Geometry: final body of the model. Coordinates: model frame, mm. Coordinates: 2 decimals unless noted, no trailing zeros. Write each loop counter-clockwise with the first axis right and the second up, starting at its lowest first coordinate (ties: lowest second). Pieces come first, ordered by that corner, then holes. Notation, with made-up numbers: (45, 23) - (104, 23) arc R17 ccw to (104, 52) - close; hole circle Ø1 at (65.25, -31.5). An arc over 180 degrees is marked (long way). Answer as a JSON object with one key per item and string values. Group by question number.
Item 1: Section C-C on y = 4.5. State how many separate pieces and enclosed holes the cut face has, and give its area (3 significant figures).
Item 2: Section D-D on z = -17. Return loops of the section in (x, y), and give its area (3 significant figures).
Item 3: Section B-B on z = 17. Return loops of the section in (x, y), and give its area (3 significant figures).
Item 4: Section A-A on x = -17. Return loops of the section in (y, z), and give its area (3 significant figures).
Item 5: First-contact query: pin 1 Ø1.5 at (x, y) = (-12.5, 1.5) entering from +Z; pin 2 Ø3 at (x, y) = (-7, 3) entering from +Z. Flat tips, straight axial feed; report the tip coordinate or a pass-through.
Item 6: Line query: line 1 along X through (y, z) = (5.25, 0); line 2 along X through (y, z) = (1.75, 17); line 3 along X through (y, z) = (4, 21). Output: solid intervals per line, ascending. Write a range as from..to.
```python
from build123d import *
from OCP.BRepFilletAPI import BRepFilletAPI_MakeFillet

# Parameters (mm, degrees)
SKETCH1_R           = 1.3
SKETCH1_R_2         = 1.4
SKETCH1_R_3         = 2.4892
BOSS_EXTRUDE1_DEPTH = 6.35
FILLET1_R1          = 3.175
FILLET1_R2          = 1.905
FILLET2_R           = 0.79375


with BuildPart() as part:
    # Sketch1 → Boss-Extrude1 (new body)
    with BuildSketch(Plane(origin=(0, 0, 0), x_dir=(1, 0, 0), z_dir=(0, 1, 0))):
        Polygon((-10.96, -11.72), (-3.2, -11.72), (-3.2, -25.4), (38.1, -25.4), (38.1, 25.4), (-38.1, 25.4), (-38.1, -25.4), (-10.96, -25.4), align=None)
        with Locations(Location((-17, -17, 0), (0, 0, 270))):
            Circle(SKETCH1_R, mode=Mode.SUBTRACT)
        with Locations(Location((-14, -14, 0), (0, 0, 270))):
            Circle(SKETCH1_R_2, mode=Mode.SUBTRACT)
        with Locations(Location((17, -17, 0), (0, 0, 270))):
            Circle(SKETCH1_R, mode=Mode.SUBTRACT)
        with Locations(Location((14, -14, 0), (0, 0, 270))):
            Circle(SKETCH1_R_2, mode=Mode.SUBTRACT)
        with Locations(Location((-14, 14, 0), (0, 0, 270))):
            Circle(SKETCH1_R_2, mode=Mode.SUBTRACT)
        with Locations(Location((-17, 17, 0), (0, 0, 270))):
            Circle(SKETCH1_R, mode=Mode.SUBTRACT)
        with Locations(Location((14, 14, 0), (0, 0, 270))):
            Circle(SKETCH1_R_2, mode=Mode.SUBTRACT)
        with Locations(Location((17, 17, 0), (0, 0, 270))):
            Circle(SKETCH1_R, mode=Mode.SUBTRACT)
        with Locations(Location((-31.75, 0, 0), (0, 0, 270))):
            Circle(SKETCH1_R_3, mode=Mode.SUBTRACT)
        with Locations(Location((31.75, -12.7, 0), (0, 0, 270))):
            Circle(SKETCH1_R_3, mode=Mode.SUBTRACT)
        with Locations(Location((31.75, 0, 0), (0, 0, 270))):
            Circle(SKETCH1_R_3, mode=Mode.SUBTRACT)
        with Locations(Location((-31.75, 12.7, 0), (0, 0, 270))):
            Circle(SKETCH1_R_3, mode=Mode.SUBTRACT)
        with Locations(Location((31.75, 12.7, 0), (0, 0, 270))):
            Circle(SKETCH1_R_3, mode=Mode.SUBTRACT)
        with Locations(Location((-31.75, -12.7, 0), (0, 0, 270))):
            Circle(SKETCH1_R_3, mode=Mode.SUBTRACT)
    extrude(amount=BOSS_EXTRUDE1_DEPTH)

    # Fillet1: one fillet with a radius per group of edges: ONE call of the kernel's fillet builder (fillet() takes one radius for all edges)
    fillet1_edges_1 = [part.edges().sort_by_distance(p)[0] for p in [
        (-38.1, 3.175, 25.4),
        (38.1, 3.175, 25.4),
        (38.1, 3.175, -25.4),
        (-38.1, 3.175, -25.4),
        (-10.96, 3.175, 25.4),
        (-3.2, 3.175, 25.4),
    ]]
    fillet1_edges_2 = [part.edges().sort_by_distance(p)[0] for p in [
        (-10.96, 3.175, 11.72),
        (-3.2, 3.175, 11.72),
    ]]
    fillet1 = BRepFilletAPI_MakeFillet(part.part.solid().wrapped)
    for e in fillet1_edges_1:
        fillet1.Add(FILLET1_R1, e.wrapped)
    for e in fillet1_edges_2:
        fillet1.Add(FILLET1_R2, e.wrapped)
    add(Compound.cast(fillet1.Shape()), mode=Mode.REPLACE)

    # Fillet2
    fillet2_edges = [part.edges().sort_by_distance(p)[0] for p in [
        (-10.402038418, 0, 12.277961582),
        (-10.402038418, 6.35, 12.277961582),
        (-3.2, 0, 17.925),
        (-3.2, 6.35, 17.925),
        (-7.08, 0, 11.72),
        (-7.08, 6.35, 11.72),
        (-10.96, 0, 17.925),
        (-10.96, 6.35, 17.925),
        (17.45, 0, 25.4),
        (17.45, 6.35, 25.4),
        (-24.53, 0, 25.4),
        (-38.1, 0, 0),
        (0, 0, -25.4),
        (38.1, 0, 0),
        (-37.17006403, 0, 24.47006403),
        (37.17006403, 0, 24.47006403),
        (37.17006403, 0, -24.47006403),
        (-37.17006403, 0, -24.47006403),
        (-11.88993597, 0, 24.47006403),
        (-2.27006403, 0, 24.47006403),
        (38.1, 6.35, 0),
        (0, 6.35, -25.4),
        (-38.1, 6.35, 0),
        (-24.53, 6.35, 25.4),
        (-37.17006403, 6.35, 24.47006403),
        (37.17006403, 6.35, 24.47006403),
        (37.17006403, 6.35, -24.47006403),
        (-37.17006403, 6.35, -24.47006403),
        (-11.88993597, 6.35, 24.47006403),
        (-2.27006403, 6.35, 24.47006403),
        (-3.757961582, 0, 12.277961582),
        (-3.757961582, 6.35, 12.277961582),
    ]]
    fillet(fillet2_edges, radius=FILLET2_R)


solid = part.part
```
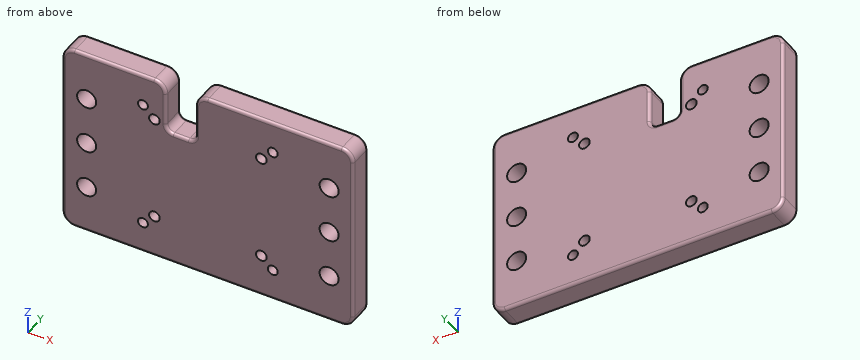
Checks:
{
 "1": {"separate pieces": "1", "enclosed holes": "14", "area": "3,590 mm^2"},
 "2": {"outline": "(-38.1, 0.79) arc R0.79 ccw to (-37.31, 0) - (-18.3, 0) - (-18.3, 6.35) - (-37.31, 6.35) arc R0.79 ccw to (-38.1, 5.56) - close; (-15.7, 0) - (15.7, 0) - (15.7, 6.35) - (-15.7, 6.35) - close; (18.3, 0) - (37.31, 0) arc R0.79 ccw to (38.1, 0.79) - (38.1, 5.56) arc R0.79 ccw to (37.31, 6.35) - (18.3, 6.35) - close", "area": "450 mm^2"},
 "3": {"outline": "(-38.1, 0.79) arc R0.79 ccw to (-37.31, 0) - (-18.3, 0) - (-18.3, 6.35) - (-37.31, 6.35) arc R0.79 ccw to (-38.1, 5.56) - close; (-15.7, 0) - (-11.75, 0) arc R0.79 ccw to (-10.96, 0.79) - (-10.96, 5.56) arc R0.79 ccw to (-11.75, 6.35) - (-15.7, 6.35) - close; (-3.2, 0.79) arc R0.79 ccw to (-2.41, 0) - (15.7, 0) - (15.7, 6.35) - (-2.41, 6.35) arc R0.79 ccw to (-3.2, 5.56) - close; (18.3, 0) - (37.31, 0) arc R0.79 ccw to (38.1, 0.79) - (38.1, 5.56) arc R0.79 ccw to (37.31, 6.35) - (18.3, 6.35) - close", "area": "400 mm^2"},
 "4": {"outline": "(0, -24.61) arc R0.79 ccw to (0.79, -25.4) - (5.56, -25.4) arc R0.79 ccw to (6.35, -24.61) - (6.35, -18.3) - (0, -18.3) - close; (0, -15.7) - (6.35, -15.7) - (6.35, 15.7) - (0, 15.7) - close; (0, 18.3) - (6.35, 18.3) - (6.35, 24.61) arc R0.79 ccw to (5.56, 25.4) - (0.79, 25.4) arc R0.79 ccw to (0, 24.61) - close", "area": "289 mm^2"},
 "5": {"pin 1": "z = 25.27", "pin 2": "z = 11.72"},
 "6": {"line 1": "-38.1..-34.24, -29.26..29.26, 34.24..38.1", "line 2": "-38.1..-18.3, -15.7..-10.96, -3.2..15.7, 18.3..38.1", "line 3": "-38.1..-10.96, -3.2..38.1"}
}
